Could you check a few things on this model? Use its own coordinates, in mm. Face numbers are marked on the shaded views. A direction names the side the tool comes from. Give positions to 0.01 mm unless a question says otherwise; leave off trailing zeros. Order: outer loops, then holes, each group sorted by start corner. A loop starts at its lowest first (then second) coordinate and runs counter-clockwise, first axis right, second up. Notation, with made-up numbers: M 32.25,-29.5 L 54.25,-29.5 A10 cw 54.25,-10.5 Z; hole C 12.25,-37 d10. An arc over 180 degrees is marked long. Answer in a Markdown table with one row per item. Add a question column.
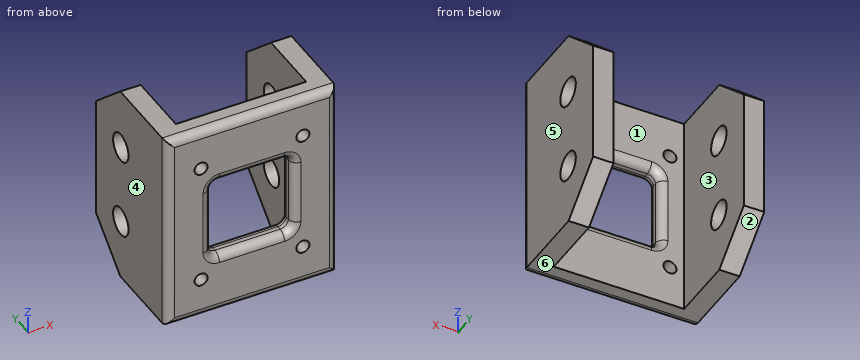
```python
from build123d import *

# Parameters (mm, degrees)
SKETCH1_W           = 63.5
SKETCH1_H           = 6.35
BOSS_EXTRUDE1_DEPTH = 53.34
BOSS_EXTRUDE2_DEPTH = 6.35
CUT_EXTRUDE1_REACH  = 94.454
SKETCH11_R          = 4.445
FILLET1_R           = 2.54
CUT_EXTRUDE2_REACH  = 94.454
SKETCH19_R          = 2.032
CUT_EXTRUDE3_DEPTH  = 6.35
FILLET2_R           = 2.54


with BuildPart() as part:
    # Sketch1 → Boss-Extrude1 (new body)
    with BuildSketch(Plane(origin=(0, 0, 0), x_dir=(0, 0, -1), z_dir=(1, 0, 0))):
        with Locations((31.75, 3.175)):
            Rectangle(SKETCH1_W, SKETCH1_H)
    extrude(amount=-BOSS_EXTRUDE1_DEPTH)

    # Sketch2 → Boss-Extrude2 (add)
    with BuildSketch(Plane(origin=(0, 0, 0), x_dir=(0, 0, -1), z_dir=(1, 0, 0))):
        Polygon((0, 6.35), (0, 26.67), (12.7, 40.869031657), (50.8, 40.869031657), (63.5, 26.67), (63.5, 6.35), align=None)
    boss_extrude2 = extrude(amount=-BOSS_EXTRUDE2_DEPTH)

    # Sketch11 → Cut-Extrude1 (cut, up to next)
    with BuildSketch(Plane(origin=(0, 0, 0), x_dir=(0, 0, -1), z_dir=(1, 0, 0)), mode=Mode.PRIVATE) as cut_extrude1_sk1:
        with Locations((19.05, 26.391031657)):
            Circle(SKETCH11_R)
    cut_extrude1_tool1 = extrude(cut_extrude1_sk1.sketch, amount=-CUT_EXTRUDE1_REACH, mode=Mode.PRIVATE) & part.part
    # Sketch11 → Cut-Extrude1 (cut, up to next)
    with BuildSketch(Plane(origin=(0, 0, 0), x_dir=(0, 0, -1), z_dir=(1, 0, 0)), mode=Mode.PRIVATE) as cut_extrude1_sk2:
        with Locations((44.45, 26.391031657)):
            Circle(SKETCH11_R)
    cut_extrude1_tool2 = extrude(cut_extrude1_sk2.sketch, amount=-CUT_EXTRUDE1_REACH, mode=Mode.PRIVATE) & part.part
    cut_extrude1_1 = cut_extrude1_tool1.solids().sort_by_distance((0, 26.391032, -19.05))[0]
    add(cut_extrude1_1, mode=Mode.SUBTRACT)
    cut_extrude1_2 = cut_extrude1_tool2.solids().sort_by_distance((0, 26.391032, -44.45))[0]
    add(cut_extrude1_2, mode=Mode.SUBTRACT)
    cut_extrude1 = cut_extrude1_1 + cut_extrude1_2  # Cut-Extrude1 as one shape, for the pattern or mirror that repeats it

    # Fillet1
    fillet1_edges = [part.edges().sort_by_distance(p)[0] for p in [
        (0, 0, -31.75),
        (-53.34, 0, -31.75),
        (-26.67, 0, -63.5),
        (-26.67, 0, 0),
    ]]
    fillet(fillet1_edges, radius=FILLET1_R)

    # Sketch19 → Cut-Extrude2 (cut, up to next)
    with BuildSketch(Plane.XZ, mode=Mode.PRIVATE) as cut_extrude2_sk1:
        with Locations(Location((-10.795, -50.8, 0), (0, 0, 270))):
            Circle(SKETCH19_R)
    cut_extrude2_tool1 = extrude(cut_extrude2_sk1.sketch, amount=-CUT_EXTRUDE2_REACH, mode=Mode.PRIVATE) & part.part
    # Sketch19 → Cut-Extrude2 (cut, up to next)
    with BuildSketch(Plane.XZ, mode=Mode.PRIVATE) as cut_extrude2_sk2:
        with Locations(Location((-42.545, -50.8, 0), (0, 0, 270))):
            Circle(SKETCH19_R)
    cut_extrude2_tool2 = extrude(cut_extrude2_sk2.sketch, amount=-CUT_EXTRUDE2_REACH, mode=Mode.PRIVATE) & part.part
    # Sketch19 → Cut-Extrude2 (cut, up to next)
    with BuildSketch(Plane.XZ, mode=Mode.PRIVATE) as cut_extrude2_sk3:
        with Locations(Location((-42.545, -12.7, 0), (0, 0, 270))):
            Circle(SKETCH19_R)
    cut_extrude2_tool3 = extrude(cut_extrude2_sk3.sketch, amount=-CUT_EXTRUDE2_REACH, mode=Mode.PRIVATE) & part.part
    # Sketch19 → Cut-Extrude2 (cut, up to next)
    with BuildSketch(Plane.XZ, mode=Mode.PRIVATE) as cut_extrude2_sk4:
        with Locations(Location((-10.795, -12.7, 0), (0, 0, 270))):
            Circle(SKETCH19_R)
    cut_extrude2_tool4 = extrude(cut_extrude2_sk4.sketch, amount=-CUT_EXTRUDE2_REACH, mode=Mode.PRIVATE) & part.part
    add(cut_extrude2_tool1.solids().sort_by_distance((-10.795, 0, -50.8))[0], mode=Mode.SUBTRACT)
    add(cut_extrude2_tool2.solids().sort_by_distance((-42.545, 0, -50.8))[0], mode=Mode.SUBTRACT)
    add(cut_extrude2_tool3.solids().sort_by_distance((-42.545, 0, -12.7))[0], mode=Mode.SUBTRACT)
    add(cut_extrude2_tool4.solids().sort_by_distance((-10.795, 0, -12.7))[0], mode=Mode.SUBTRACT)

    # Mirror1: Boss-Extrude2, Cut-Extrude1 across plane
    add(boss_extrude2.mirror(Plane(origin=(-26.67, 0, 0), x_dir=(0, 0, 1), z_dir=(1, 0, 0))))
    add(cut_extrude1.mirror(Plane(origin=(-26.67, 0, 0), x_dir=(0, 0, 1), z_dir=(1, 0, 0))), mode=Mode.SUBTRACT)

    # Sketch20 → Cut-Extrude3 (cut)
    with BuildSketch(Plane.XZ):
        with BuildLine():
            Line((-16.51, -19.05), (-36.83, -19.05))
            ThreePointArc((-36.83, -19.05), (-38.626051224, -19.793948776), (-39.37, -21.59))
            Line((-39.37, -21.59), (-39.37, -41.91))
            ThreePointArc((-39.37, -41.91), (-38.626051224, -43.706051224), (-36.83, -44.45))
            Line((-36.83, -44.45), (-16.51, -44.45))
            ThreePointArc((-16.51, -44.45), (-14.713948776, -43.706051224), (-13.97, -41.91))
            Line((-13.97, -41.91), (-13.97, -21.59))
            ThreePointArc((-13.97, -21.59), (-14.713948776, -19.793948776), (-16.51, -19.05))
        make_face()
    extrude(amount=-CUT_EXTRUDE3_DEPTH, mode=Mode.SUBTRACT)

    # Fillet2
    fillet2_edges = [part.edges().sort_by_distance(p)[0] for p in [
        (-38.626051224, 0, -43.706051224),
        (-26.67, 0, -44.45),
        (-14.713948776, 0, -43.706051224),
        (-13.97, 0, -31.75),
        (-14.713948776, 0, -19.793948776),
        (-26.67, 0, -19.05),
        (-38.626051224, 0, -19.793948776),
        (-39.37, 0, -31.75),
        (-26.67, 6.35, -44.45),
        (-14.713948776, 6.35, -43.706051224),
        (-13.97, 6.35, -31.75),
        (-14.713948776, 6.35, -19.793948776),
        (-26.67, 6.35, -19.05),
        (-38.626051224, 6.35, -19.793948776),
        (-39.37, 6.35, -31.75),
        (-38.626051224, 6.35, -43.706051224),
    ]]
    fillet(fillet2_edges, radius=FILLET2_R)


solid = part.part
```
1. If I drill on line 1 along X through (y, z) = (4, -50); line 2 along X through (y, z) = (3, -12); line 3 along X through (y, z) = (17, -14.5), over which ranges is the centre line in solid material (lowest first)? Write a range as [from, to].
2. Suppose I cut it at B-B on x = -34. List the corners of the cut face in (y, z) for me, plus the area to 3 significant figures.
3. Thinking about a two-plate mould opening in X: for the marked faces 3, 4, 5 and 6, which applies, pulls with the +X half, pulls with the -X half, needs draft (parallel to the pull), parting line crosses it, or undercut?
4. Suppose I cut it at D-D on y = 36.5. List the corners of the cut face in (x, z) for me, plus the area to 3 significant figures.
5. Will these pins go through, and if not, where does the flat tip stop? P1, Ø5.5, axis at x = -42.545, z = -12.7, coming from the +Y side; P2, Ø12, axis at x = -30.5, z = -39, coming from the +Y side.
6. Suppose I cut it at C-C on z = -20. Count the separate pieces of the cut face and the enclosed holes in it, plus the area to 3 significant figures.
7. Suppose I cut it at A-A on y = 19. List the corners of the cut face in (x, z) for me.
8. For the marked faces 1 and 2, which set-ups out of +Z, -Z, +X, -X, +Y, -Y let a thin tool reach every point of the face, with its end or its side?
Findings below:
| question | item | result |
|---|---|---|
| 1 | line 1 | [-53.34, -44.41], [-40.68, -12.66], [-8.93, 0] |
| 1 | line 2 | [-53.34, -44.45], [-40.64, -12.7], [-8.89, 0] |
| 1 | line 3 | [-53.34, -46.99], [-6.35, 0] |
| 2 | outline | M 0,-60.96 A2.54 ccw 2.54,-63.5 L 6.35,-63.5 L 6.35,-46.99 A2.54 ccw 3.81,-44.45 L 2.54,-44.45 A2.54 ccw 0,-46.99 Z; M 0,-16.51 A2.54 ccw 2.54,-19.05 L 3.81,-19.05 A2.54 ccw 6.35,-16.51 L 6.35,0 L 2.54,0 A2.54 ccw 0,-2.54 Z |
| 2 | area | 234 mm2 |
| 3 | face 3 | undercut |
| 3 | face 4 | pulls with the -X half |
| 3 | face 5 | pulls with the +X half |
| 3 | face 6 | needs draft |
| 4 | outline | M -53.34,-54.71 L -46.99,-54.71 L -46.99,-8.79 L -53.34,-8.79 Z; M -6.35,-54.71 L 0,-54.71 L 0,-8.79 L -6.35,-8.79 Z |
| 4 | area | 583 mm2 |
| 5 | P1 | y = 6.35 |
| 5 | P2 | y = 5.39 |
| 6 | separate pieces | 4 |
| 6 | enclosed holes | 0 |
| 6 | area | 503 mm2 |
| 7 | outline | M -53.34,-63.5 L -46.99,-63.5 L -46.99,0 L -53.34,0 Z; M -6.35,-63.5 L 0,-63.5 L 0,0 L -6.35,0 Z |
| 8 | face 1 | +Z, -Z, +Y |
| 8 | face 2 | -Z, +X, -X, +Y |
